Here's how the part is built. I have some questions about the finished solid (model axes, mm). Face numbers are marked on the shaded views. Coordinates: 2 decimals unless noted, no trailing zeros. Loops run counter-clockwise (first coordinate to the right, second up) from the corner with the lowest first, then second, coordinate; pieces in that order, holes last. Notation, with made-up numbers: (34.25, 30) -> (44.25, 30) arc R28 cw to (44.25, 62) -> close; hole circle Ø1 at (48.5, 54). An arc over 180 degrees is marked (long way). Answer as a JSON object with one key per item and string values. Group by question number.
Q1. Thinking about a two-plate mould opening in Y: for the marked faces 1, 2, 3 and 4, which applies, released by +Y, released by -Y, zero draft, split by the parting line, or undercut?
Q2. I'm going to push flat-ended pins straight in: pin 1 (1 mm diameter, centred on y = -19, z = 6, fed in from +X); pin 2 (10 mm diameter, centred on x = 40.5, y = 16.5, fed in from -Z). Where does each tip first touch, or does it pass through?
Q3. I want a section at C-C on y = 3. Write out the boundary of the cut face in (x, z) (3 decimals).
Q4. I want a section at B-B on z = 6. Write out the boundary of the cut face in (x, y), then the cut area to 3 significant figures.
Q5. I need wall thicknesses on line 1 (Y direction, x = 12.5, z = 3.5); line 2 (X direction, y = -3.5, z = 7.25); line 3 (Y direction, x = -31.5, z = 6). Which ranges of each line are inside material? Lowest first, please.
Q6. I want a section at D-D on x = 12.7. Write out the boundary of the cut face in (y, z) (3 decimals).
Q7. I want a section at A-A on x = 44.45. Write out the boundary of the cut face in (y, z) (3 decimals), then the cut area to 3 significant figures.
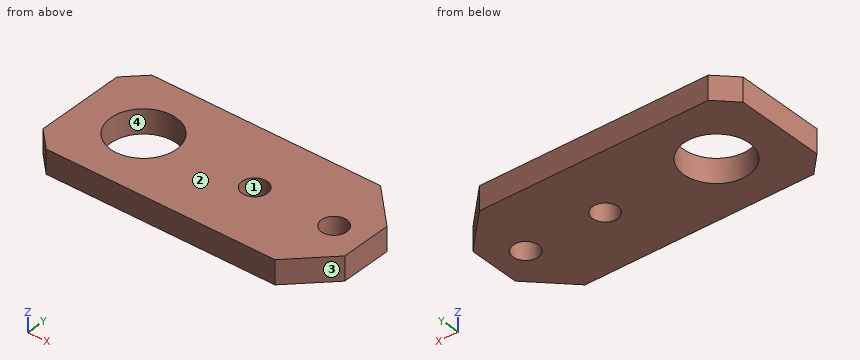
```python
from build123d import *

# Parameters (mm, degrees)
SKETCH1_W               = 114.3
SKETCH1_H               = 50.8
BOSS_EXTRUDE1_DEPTH     = 9.525
F_3_8_CLEARANCE_HOLE1_D = 10.0838
F_1_CLEARANCE_HOLE1_D   = 26.19248
CHAMFER1_SIZE           = 7.62
CHAMFER2_SIZE           = 15.24


with BuildPart() as part:
    # Sketch1 → Boss-Extrude1 (new body)
    with BuildSketch(Plane.XY):
        Rectangle(SKETCH1_W, SKETCH1_H)
    extrude(amount=BOSS_EXTRUDE1_DEPTH)

    # 3/8 Clearance Hole1 (through all)
    with Locations(Plane.XY.offset(9.525)):
        with Locations((44.45, 0), (12.7, 0)):
            Hole(F_3_8_CLEARANCE_HOLE1_D / 2)

    # 1 Clearance Hole1 (through all)
    with Locations(Plane.XY.offset(9.525)):
        with Locations((-31.75, 0)):
            Hole(F_1_CLEARANCE_HOLE1_D / 2)

    # Chamfer1
    chamfer1_edges = [part.edges().sort_by_distance(p)[0] for p in [
        (-57.15, -25.4, 4.7625),
        (-57.15, 25.4, 4.7625),
    ]]
    chamfer(chamfer1_edges, length=CHAMFER1_SIZE)

    # Chamfer2
    chamfer2_edges = [part.edges().sort_by_distance(p)[0] for p in [
        (57.15, -25.4, 4.7625),
        (57.15, 25.4, 4.7625),
    ]]
    chamfer(chamfer2_edges, length=CHAMFER2_SIZE)


solid = part.part
```
Result set:
{
 "1": {"face 1": "undercut", "face 2": "zero draft", "face 3": "released by -Y", "face 4": "undercut"},
 "2": {"pin 1": "stops at x = 48.81", "pin 2": "stops at z = 0"},
 "3": {"outline": "(-57.15, 0) -> (-44.498, 0) -> (-44.498, 9.525) -> (-57.15, 9.525) -> close; (-19.002, 0) -> (8.648, 0) -> (8.648, 9.525) -> (-19.002, 9.525) -> close; (16.752, 0) -> (40.398, 0) -> (40.398, 9.525) -> (16.752, 9.525) -> close; (48.502, 0) -> (57.15, 0) -> (57.15, 9.525) -> (48.502, 9.525) -> close"},
 "4": {"outline": "(-57.15, -17.78) -> (-49.53, -25.4) -> (41.91, -25.4) -> (57.15, -10.16) -> (57.15, 10.16) -> (41.91, 25.4) -> (-49.53, 25.4) -> (-57.15, 17.78) -> close; hole circle Ø26.19 at (-31.75, 0); hole circle Ø10.08 at (12.7, 0); hole circle Ø10.08 at (44.45, 0)", "area": "4,820 mm²"},
 "5": {"line 1": "y = -25.4 to -5.04, 5.04 to 25.4", "line 2": "x = -57.15 to -44.37, -19.13 to 9.07, 16.33 to 40.82, 48.08 to 57.15", "line 3": "y = -25.4 to -13.09, 13.09 to 25.4"},
 "6": {"outline": "(-25.4, 0) -> (-5.042, 0) -> (-5.042, 9.525) -> (-25.4, 9.525) -> close; (5.042, 0) -> (25.4, 0) -> (25.4, 9.525) -> (5.042, 9.525) -> close"},
 "7": {"outline": "(-22.86, 0) -> (-5.042, 0) -> (-5.042, 9.525) -> (-22.86, 9.525) -> close; (5.042, 0) -> (22.86, 0) -> (22.86, 9.525) -> (5.042, 9.525) -> close", "area": "339 mm²"}
}
